Could you check a few things on this drawing? It's one solid part, dimensions in mm from its lowest x, y, z. A direction names the side the tool comes from. Round coordinates to 2 decimals unless told otherwise and drop trailing zeros. Write each loop counter-clockwise with the first axis right and the second up, starting at its lowest first coordinate (ties: lowest second). Pieces come first, ordered by that corner, then holes. Notation, with made-up numbers: (80, -30.75) -> (87, -30.75) arc R21 cw to (87, -15.75) -> close; hole circle Ø4 at (-12, 62.25). An arc over 180 degrees is marked (long way). Answer in a Markdown table with one row per item.
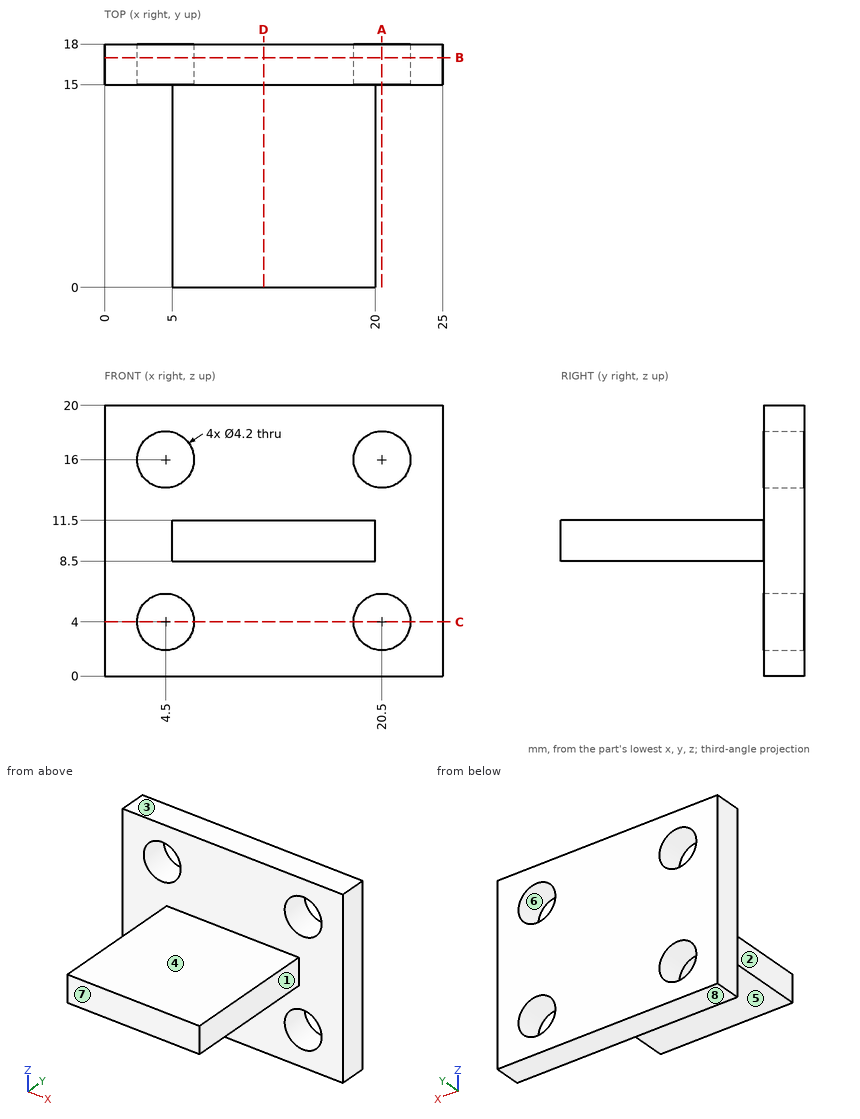
1) Imagine slicing it at B-B, the plane y = 17. Please give me the cut outline in (x, z).
Findings:
| item | result |
|---|---|
| outline | (0, 0) -> (25, 0) -> (25, 20) -> (0, 20) -> close; hole circle Ø4.2 at (4.5, 4); hole circle Ø4.2 at (4.5, 16); hole circle Ø4.2 at (20.5, 4); hole circle Ø4.2 at (20.5, 16) |
2) Imagine slicing it at C-C, the plane z = 4. Please give me the cut outline in (x, y).
Findings:
| item | result |
|---|---|
| outline | (0, 15) -> (2.4, 15) -> (2.4, 18) -> (0, 18) -> close; (6.6, 15) -> (18.4, 15) -> (18.4, 18) -> (6.6, 18) -> close; (22.6, 15) -> (25, 15) -> (25, 18) -> (22.6, 18) -> close |
3) Thinking about a two-plate mould opening in Z: for the marked faces 6, 7 and 8, which applies, +Z half, -Z half, draft (parallel to the pull), parting line (faces both ways), or undercut?
Findings:
| item | result |
|---|---|
| face 6 | undercut |
| face 7 | draft |
| face 8 | -Z half |
4) Imagine slicing it at D-D, the plane x = 11.75. Please give me the cut outline in (y, z), plus the area to 3 significant figures.
Findings:
| item | result |
|---|---|
| outline | (0, 8.5) -> (15, 8.5) -> (15, 0) -> (18, 0) -> (18, 20) -> (15, 20) -> (15, 11.5) -> (0, 11.5) -> close |
| area | 105 mm^2 |
5) Please list where these lines run through material, in increasing order: line 1 (X direction, y = 17.4, z = 4); line 2 (Z direction, x = 20.5, y = 16.4); line 3 (X direction, y = 15.5, z = 14.5).
Findings:
| item | result |
|---|---|
| line 1 | x = 0 to 2.4, 6.6 to 18.4, 22.6 to 25 |
| line 2 | z = 0 to 1.9, 6.1 to 13.9, 18.1 to 20 |
| line 3 | x = 0 to 3.03, 5.97 to 19.03, 21.97 to 25 |
6) Imagine slicing it at A-A, the plane x = 20.5. Please give me the cut outline in (y, z).
Findings:
| item | result |
|---|---|
| outline | (15, 0) -> (18, 0) -> (18, 1.9) -> (15, 1.9) -> close; (15, 6.1) -> (18, 6.1) -> (18, 13.9) -> (15, 13.9) -> close; (15, 18.1) -> (18, 18.1) -> (18, 20) -> (15, 20) -> close |
7) For the marked faces 1, 2, 3, 4 and 5, which set-ups out of +Z, -Z, +X, -X, +Y, -Y let a thin tool reach every point of the face, with its end or its side?
Findings:
| item | result |
|---|---|
| face 1 | +Z, -Z, +X, -Y |
| face 2 | +Z, -Z, -X, -Y |
| face 3 | +Z, +X, -X, +Y, -Y |
| face 4 | +Z, +X, -X, -Y |
| face 5 | -Z, +X, -X, -Y |
8) For pin 1 (6.5 mm diameter, centred on x = 4.5, z = 16, fed in from -Y); pin 2 (1.5 mm diameter, centred on y = 4, z = 9.5, fed in from +X); pin 3 (4 mm diameter, centred on x = 4.5, z = 4, fed in from -Y); pin 4 (0.9 mm diameter, centred on y = 6.5, z = 10, fed in from -X), each with a flat end and sliding along its axis, tell me the tip position at first contact or that it passes through.
Findings:
| item | result |
|---|---|
| pin 1 | stops at y = 15 |
| pin 2 | stops at x = 20 |
| pin 3 | passes through |
| pin 4 | stops at x = 5 |
